Source: CAD feature listing. Evaluate the final solid. Frame: model axes, mm. Face numbers are marked on the shaded views. A direction names the side the tool comes from. Give positions to 0.01 mm unless a question says otherwise; leave off trailing zeros. Order: outer loops, then holes, each group sorted by start corner. A loop starts at its lowest first (then second) coordinate and runs counter-clockwise, first axis right, second up. Notation, with made-up numbers: (2.25, -18) - (44.25, -18) arc R25 ccw to (44.25, 4) - close; hole circle Ø9 at (58.25, -5.5). An arc over 180 degrees is marked (long way). One line per item, written item: value. Start each with the question number.
from build123d import *

# Parameters (mm, degrees)
SKETCH1_R           = 1.425
BOSS_EXTRUDE1_DEPTH = 13
SKETCH2_W           = 13
SKETCH2_H           = 13
SKETCH2_R           = 3.075
BOSS_EXTRUDE2_DEPTH = 12
BOSS_EXTRUDE3_REACH = 28.636
SKETCH5_R           = 1.425
CUT_EXTRUDE1_DEPTH  = 12
FILLET2_R           = 1


with BuildPart() as part:
    # Sketch1 → Boss-Extrude1 (new body)
    with BuildSketch(Plane(origin=(0, 0, 0), x_dir=(1, 0, 0), z_dir=(0, 1, 0))):
        Polygon((0, -3.75277675), (3.25, -1.876388375), (3.25, 1.876388375), (0, 3.75277675), (-3.25, 1.876388375), (-3.25, -1.876388375), align=None)
        with Locations(Location((0, 0, 0), (0, 0, 90))):
            Circle(SKETCH1_R, mode=Mode.SUBTRACT)
    extrude(amount=BOSS_EXTRUDE1_DEPTH)

    # Sketch2 → Boss-Extrude2 (add)
    with BuildSketch(Plane(origin=(0, 13, 0), x_dir=(1, 0, 0), z_dir=(0, 1, 0))):
        Rectangle(SKETCH2_W, SKETCH2_H)
        with Locations(Location((0, 0, 0), (0, 0, 270))):
            Circle(SKETCH2_R, mode=Mode.SUBTRACT)
    extrude(amount=BOSS_EXTRUDE2_DEPTH)

    # Sketch3 → Boss-Extrude3 (add, up to next)
    with BuildSketch(Plane(origin=(0, 25, 0), x_dir=(1, 0, 0), z_dir=(0, 1, 0)), mode=Mode.PRIVATE) as boss_extrude3_sk1:
        with BuildLine():
            Line((-1.516575089, 2.675), (1.516575089, 2.675))
            ThreePointArc((1.516575089, 2.675), (0, 3.075), (-1.516575089, 2.675))
        make_face()
    boss_extrude3_tool1 = extrude(boss_extrude3_sk1.sketch, amount=-BOSS_EXTRUDE3_REACH, mode=Mode.PRIVATE) - part.part
    add(boss_extrude3_tool1.solids().sort_by_distance((0, 25, -2.835927))[0])

    # Sketch5 → Cut-Extrude1 (cut)
    with BuildSketch(Plane.XY.offset(-2.675)):
        with Locations((0, 20)):
            Circle(SKETCH5_R)
    extrude(amount=-CUT_EXTRUDE1_DEPTH, mode=Mode.SUBTRACT)

    # Fillet2
    fillet2_edges = [part.edges().sort_by_distance(p)[0] for p in [
        (-6.5, 19, -6.5),
        (-6.5, 19, 6.5),
        (6.5, 19, 6.5),
        (6.5, 19, -6.5),
    ]]
    fillet(fillet2_edges, radius=FILLET2_R)

    # Sketch8 → Revolve1 (revolve)
    with BuildSketch(Plane(origin=(0, 0, 0), x_dir=(0, 0, -1), z_dir=(1, 0, 0))):
        Polygon((0, 13), (-3.75277675, 13), (-6.25277675, 13), (-3.75277675, 11), (0, 11), align=None)
    revolve(axis=Axis((0, -1000, 0), (0, 1, 0)))


solid = part.part
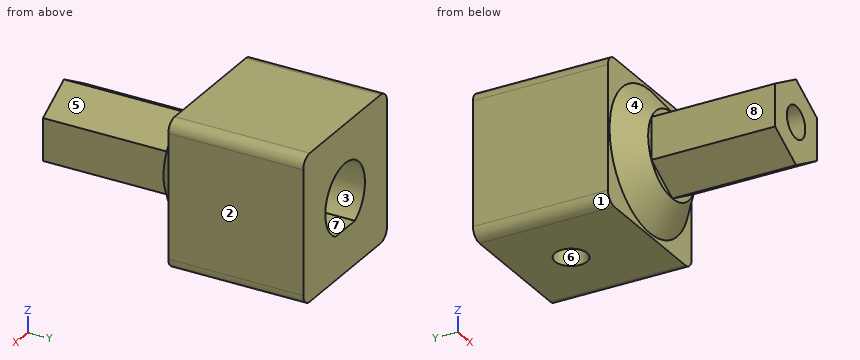
1. Draft query along Z for the marked faces 1, 2, 3 and 4. Return one class per face: pulls with the +Z half, pulls with the -Z half, needs draft (parallel to the pull), parting line crosses it, or undercut.
2. Section A-A on y = 7. Return the cut outline in (x, z) (3 decimals).
3. Section B-B on z = 0. Return the cut outline in (x, y) (3 decimals), then the cut area to 3 significant figures.
4. Ray query, L1, parallel to X at y = 20, z = 0 (3 decimals); L2, parallel to X at y = 3, z = 0 (3 decimals); L3, parallel to Y at x = 2.5, z = -2.5. Return the intervals inside material, ascending.
5. Set-up query: the marked faces 5, 6, 7 and 8. Return all of +Z, -Z, +X, -X, +Y, -Y with unobstructed straight access to the full face (end or side cutting, diameter ignored); none if empty.
6. Section C-C on y = 20. Return the cut outline in (x, z) (3 decimals), then the cut area to 3 significant figures.
7. Contact query for flat-ended pins moving along their axis: pin 1 Ø5 at (x, y) = (3, 5.5) entering from -Z; pin 2 Ø1.1 at (y, z) = (5, 0) entering from +X; pin 3 Ø3.5 at (x, z) = (0, 0) entering from +Y; pin 4 Ø2 at (x, y) = (-5, 7) entering from +Z. Output: stop coordinate, or through.
Data:
1. face 1: pulls with the -Z half
1. face 2: needs draft
1. face 3: undercut
1. face 4: parting line crosses it
2. outline: (-3.25, -1.876) - (0, -3.753) - (3.25, -1.876) - (3.25, 1.876) - (0, 3.753) - (-3.25, 1.876) - close; hole circle Ø2.85 at (0, 0)
3. outline: (-6.5, 13) - (-6.253, 13) - (-3.753, 11) - (-3.25, 11) - (-3.25, 0) - (-1.425, 0) - (-1.425, 11) - (1.425, 11) - (1.425, 0) - (3.25, 0) - (3.25, 11) - (3.753, 11) - (6.253, 13) - (6.5, 13) - (6.5, 25) - (3.075, 25) - (3.075, 13) - (-3.075, 13) - (-3.075, 25) - (-6.5, 25) - close
3. area: 142 mm2
4. L1: x = -6.5 to -3.075, 3.075 to 6.5
4. L2: x = -3.25 to -1.425, 1.425 to 3.25
4. L3: y = 11 to 25
5. face 5: +Z, +X, -Y
5. face 6: -Z
5. face 7: +Y
5. face 8: +Z, -Z, -X, -Y
6. outline: (-6.5, -5.5) arc R1 ccw to (-5.5, -6.5) - (-1.425, -6.5) - (-1.425, -2.675) - (-1.517, -2.675) arc R3.075 cw (long way) to (1.517, -2.675) - (1.425, -2.675) - (1.425, -6.5) - (5.5, -6.5) arc R1 ccw to (6.5, -5.5) - (6.5, 5.5) arc R1 ccw to (5.5, 6.5) - (-5.5, 6.5) arc R1 ccw to (-6.5, 5.5) - close
6. area: 128 mm2
7. pin 1: stops at z = -3.46
7. pin 2: stops at x = 3.25
7. pin 3: stops at y = 13
7. pin 4: passes through
